Part model, mm, in its own coordinate system. A direction names the side the tool comes from. Round coordinates to 2 decimals unless told otherwise and drop trailing zeros. Write each loop counter-clockwise with the first axis right and the second up, starting at its lowest first coordinate (ties: lowest second). Pieces come first, ordered by that corner, then holes. Notation, with made-up numbers: M -36,29.25 L -23,29.25 A13 ccw -23,39.25 Z; hole C 43,-4 d9. An arc over 180 degrees is marked long. Answer as a JSON object with one key per item and string values. Group by question number.
1. Two-plate mould, pull along X, no slides. Class faces 4 (the face through (245, 3, 75)), 5 (the face through (260, 3, 46)), 6 (the face through (128, 0, 44)), 7 (the face through (0, 5, 45)): +X half, -X half, draft (parallel to the pull), parting line (faces both ways), or undercut.
2. Band-saw the part on B-B, the plane x = 242.5. Write the cut outline in (y, z), plus the area to 3 significant figures.
3. Band-saw the part on D-D, the plane z = 84.5. Write the cut outline in (x, y).
4. Drill centre lines: line 1 (Z direction, x = 242.5, y = 3.45); line 2 (X direction, y = 8.95, z = 67.5); line 3 (X direction, y = 2, z = 30). Where is each one in solid material? Low to high. Write a range as from..to.
5. Band-saw the part on C-C, the plane y = 8.5. Write the cut outline in (x, z).
6. Band-saw the part on A-A, the plane z = 30. Write the cut outline in (x, y).
7. Drop flat-ended pins along their axis: pin 1 (3.5 mm diameter, centred on x = 72.5, z = 24, fed in from -Y); pin 2 (4.5 mm diameter, centred on x = 242.5, z = 60, fed in from -Y); pin 3 (3 mm diameter, centred on y = 8.5, z = 50, fed in from +X); pin 4 (8 mm diameter, centred on x = 242.5, z = 15, fed in from +Y). Give the stop position or say it passes through.
8. Which spindle directions (+Z, -Z, +X, -X, +Y, -Y) get a long thin tool onto all of the face, cutting with end or side? Do faces 1 (the face through (244.61, 3.04, 46.34)), 2 (the face through (24.11, 2.54, 70.28)), 3 (the face through (246, 6, 44)). Say none if no direction does.
from build123d import *

# Parameters (mm, degrees)
SKETCH_1_W          = 260
SKETCH_1_H          = 90
EXTRUDE_1_DEPTH     = 10
SKETCH_2_W          = 35
SKETCH_2_H          = 90
CUT_EXTRUDE_1_DEPTH = 4
SKETCH_3_R          = 1.5
CUT_EXTRUDE_2_DEPTH = 10
CUT_EXTRUDE_START   = -5
SKETCH_4_R          = 3.5
SKETCH_4_R_2        = 1.5
CUT_EXTRUDE_3_DEPTH = 5
SKETCH_5_R          = 2.5
CUT_EXTRUDE_4_DEPTH = 25
FILLET_1_R          = 10


with BuildPart() as part:
    # 草图1 → 凸台-拉伸1 (new body)
    with BuildSketch(Plane(origin=(0, 0, 0), x_dir=(1, 0, 0), z_dir=(0, 1, 0))):
        with Locations((130, -45)):
            Rectangle(SKETCH_1_W, SKETCH_1_H)
    extrude(amount=EXTRUDE_1_DEPTH)

    # 草图2 → 切除-拉伸1 (cut)
    with BuildSketch(Plane(origin=(0, 10, 0), x_dir=(1, 0, 0), z_dir=(0, 1, 0))):
        with Locations((242.5, -45)):
            Rectangle(SKETCH_2_W, SKETCH_2_H)
    extrude(amount=-CUT_EXTRUDE_1_DEPTH, mode=Mode.SUBTRACT)

    # 草图3 → 切除-拉伸2 (cut)
    with BuildSketch(Plane(origin=(0, 10, 0), x_dir=(1, 0, 0), z_dir=(0, 1, 0))):
        with Locations(Location((26.239488698, -22.5, 0), (0, 0, 270))):
            Circle(SKETCH_3_R)
        with Locations(Location((26.239488698, -67.5, 0), (0, 0, 270))):
            Circle(SKETCH_3_R)
        with Locations(Location((71.239488698, -67.5, 0), (0, 0, 270))):
            Circle(SKETCH_3_R)
        with Locations(Location((71.239488698, -22.5, 0), (0, 0, 270))):
            Circle(SKETCH_3_R)
    extrude(amount=-CUT_EXTRUDE_2_DEPTH, mode=Mode.SUBTRACT)

    # 草图4 → 切除-拉伸3 (cut)
    # profile 1 of 4: a face of its own
    with BuildSketch(Plane.XZ.offset(CUT_EXTRUDE_START)):
        with Locations(Location((26.239488698, 67.5, 0), (0, 0, 270))):
            Circle(SKETCH_4_R)
        with Locations(Location((26.239488698, 67.5, 0), (0, 0, 90))):
            Circle(SKETCH_4_R_2, mode=Mode.SUBTRACT)
    # profile 2 of 4: a face of its own
    with BuildSketch(Plane.XZ.offset(CUT_EXTRUDE_START)):
        with Locations(Location((26.239488698, 22.5, 0), (0, 0, 270))):
            Circle(SKETCH_4_R)
        with Locations(Location((26.239488698, 22.5, 0), (0, 0, 90))):
            Circle(SKETCH_4_R_2, mode=Mode.SUBTRACT)
    # profile 3 of 4: a face of its own
    with BuildSketch(Plane.XZ.offset(CUT_EXTRUDE_START)):
        with Locations(Location((71.239488698, 22.5, 0), (0, 0, 270))):
            Circle(SKETCH_4_R)
        with Locations(Location((71.239488698, 22.5, 0), (0, 0, 90))):
            Circle(SKETCH_4_R_2, mode=Mode.SUBTRACT)
    # profile 4 of 4: a face of its own
    with BuildSketch(Plane.XZ.offset(CUT_EXTRUDE_START)):
        with Locations(Location((71.239488698, 67.5, 0), (0, 0, 270))):
            Circle(SKETCH_4_R)
        with Locations(Location((71.239488698, 67.5, 0), (0, 0, 90))):
            Circle(SKETCH_4_R_2, mode=Mode.SUBTRACT)
    extrude(amount=CUT_EXTRUDE_3_DEPTH, mode=Mode.SUBTRACT)

    # 草图5 → 切除-拉伸4 (cut)
    with BuildSketch(Plane(origin=(0, 6, 0), x_dir=(1, 0, 0), z_dir=(0, 1, 0))):
        with Locations(Location((242.5, -45, 0), (0, 0, 270))):
            Circle(SKETCH_5_R)
        with Locations(Location((242.5, -15, 0), (0, 0, 270))):
            Circle(SKETCH_5_R)
        with Locations(Location((242.5, -75, 0), (0, 0, 270))):
            Circle(SKETCH_5_R)
        with Locations(Location((242.5, -30, 0), (0, 0, 270))):
            Circle(SKETCH_5_R)
        with Locations(Location((242.5, -60, 0), (0, 0, 270))):
            Circle(SKETCH_5_R)
    extrude(amount=-CUT_EXTRUDE_4_DEPTH, mode=Mode.SUBTRACT)

    # 圆角1
    fillet_1_edges = [part.edges().sort_by_distance(p)[0] for p in [
        (0, 5, 0),
        (0, 5, 90),
    ]]
    fillet(fillet_1_edges, radius=FILLET_1_R)


solid = part.part
Worked answers:
{
 "1": {"face 4": "undercut", "face 5": "+X half", "face 6": "draft", "face 7": "-X half"},
 "2": {"outline": "M 0,0 L 6,0 L 6,12.5 L 0,12.5 Z; M 0,17.5 L 6,17.5 L 6,27.5 L 0,27.5 Z; M 0,32.5 L 6,32.5 L 6,42.5 L 0,42.5 Z; M 0,47.5 L 6,47.5 L 6,57.5 L 0,57.5 Z; M 0,62.5 L 6,62.5 L 6,72.5 L 0,72.5 Z; M 0,77.5 L 6,77.5 L 6,90 L 0,90 Z", "area": "390 mm^2"},
 "3": {"outline": "M 1.07,0 L 260,0 L 260,6 L 225,6 L 225,10 L 1.07,10 Z"},
 "4": {"line 1": "z = 0..12.5, 17.5..27.5, 32.5..42.5, 47.5..57.5, 62.5..72.5, 77.5..90", "line 2": "x = 0..24.74, 27.74..69.74, 72.74..225", "line 3": "x = 0..240, 245..260"},
 "5": {"outline": "M 0,10 A10 ccw 10,0 L 225,0 L 225,90 L 10,90 A10 ccw 0,80 Z; hole C 26.24,22.5 d3; hole C 26.24,67.5 d3; hole C 71.24,22.5 d3; hole C 71.24,67.5 d3"},
 "6": {"outline": "M 0,0 L 240,0 L 240,6 L 225,6 L 225,10 L 0,10 Z; M 245,0 L 260,0 L 260,6 L 245,6 Z"},
 "7": {"pin 1": "stops at y = 0", "pin 2": "passes through", "pin 3": "stops at x = 225", "pin 4": "stops at y = 6"},
 "8": {"face 1": "+Y, -Y", "face 2": "-Y", "face 3": "+Z, -Z, +X, +Y"}
}
